Answer from the drawing. Dimensions are ordinates in mm from the lowest x, y and z of the part. A direction names the side the tool comes from. Give positions to 0.01 mm unless a question says otherwise; leave off trailing zeros. Order: outer loops, then holes, each group sorted by start corner. A loop starts at its lowest first (then second) coordinate and runs counter-clockwise, first axis right, second up.
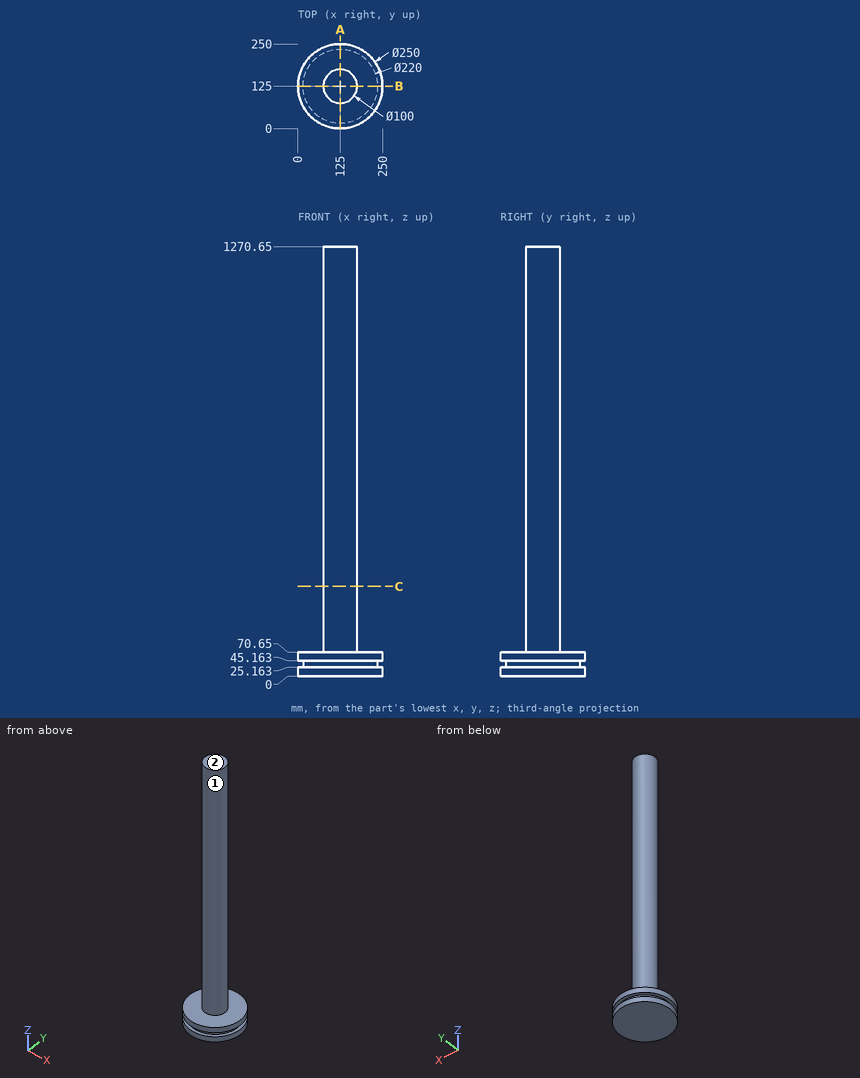
1. Given P1, Ø10, axis at x = 159, z = 618.5, coming from the -Y side; P2, Ø3, axis at x = 128, z = 224, coming from the -Y side; P3, Ø12, axis at x = 69, y = 143.5, coming from the +Z side, each flat-ended and moving along its own axis, determine where each tip first touches the part or whether it passes through.
Findings below:
P1: stops at y = 84.27
P2: stops at y = 75.02
P3: stops at z = 70.65
2. The part is cut by section A-A (x = 125). Write down the section's boundary in (y, z).
Findings below:
outline: (0, 0) - (250, 0) - (250, 25.16) - (235, 25.16) - (235, 45.16) - (250, 45.16) - (250, 70.65) - (175, 70.65) - (175, 1270.65) - (75, 1270.65) - (75, 70.65) - (0, 70.65) - (0, 45.16) - (15, 45.16) - (15, 25.16) - (0, 25.16) - close
3. Which of the six approach directions +Z, -Z, +X, -X, +Y, -Y give full straight-line access (tool end or side, diameter ignored) to the marked faces 1 and 2?
Findings below:
face 1: +Z
face 2: +Z, +X, -X, +Y, -Y
4. The part is cut by section C-C (z = 265). Write down the section's boundary in (x, y).
Findings below:
outline: circle Ø100 at (125, 125)
5. Straight lines are drawn through the part: probe 1 along Z at (x, y) = (168.5, 14); probe 2 along Z at (x, y) = (34.5, 146.5); probe 3 along X at (y, z) = (120.5, 1056.5). For each, find the intervals that lie inside material, in ascending order.
Findings below:
probe 1: z = 0 to 25.16, 45.16 to 70.65
probe 2: z = 0 to 70.65
probe 3: x = 75.2 to 174.8
